```python
from build123d import *

# Parameters (mm, degrees)
F1_DEPTH = 2.2
F2_R     = 4


with BuildPart() as f1:
    # F0 (on Front) → F1 (new body)
    with BuildSketch(Plane.XZ):
        with BuildLine():
            Line((-31, 0), (31, 0))
            Line((31, 0), (31, 11.8))
            ThreePointArc((31, 11.8), (22.8, 20), (31, 28.2))
            Line((31, 28.2), (31, 42))
            Line((31, 42), (-31, 42))
            Line((-31, 42), (-31, 28.2))
            ThreePointArc((-31, 28.2), (-22.8, 20), (-31, 11.8))
            Line((-31, 11.8), (-31, 0))
        make_face()
    extrude(amount=F1_DEPTH)

    # F2
    f2_edges = [f1.edges().sort_by_distance(p)[0] for p in [
        (-31, -1.1, 11.8),
        (31, -1.1, 11.8),
        (31, -1.1, 28.2),
        (-31, -1.1, 28.2),
    ]]
    fillet(f2_edges, radius=F2_R)


solid = f1.part
```
Geometry check sheet. Reference: the model listing, model coordinates, mm. A direction names the side the tool comes from. Round coordinates to 2 decimals unless told otherwise and drop trailing zeros. Loops run counter-clockwise (first coordinate to the right, second up) from the corner with the lowest first, then second, coordinate; pieces in that order, holes last. Notation, with made-up numbers: (79.5, 82) - (120.5, 82) arc R13 cw to (120.5, 104) - close; hole circle Ø5 at (-28, 73.5). An arc over 180 degrees is marked (long way). Write item = value, one per line. Start each with the question number.
1. Mould release check, pull along Z, two halves, no side actions. Record for faces 1 (the face through (-30.279, -1.115, 29.235)), 2 (the face through (0, -1, 0)), 3 (the face through (-31, -1, 37)): released by +Z, released by -Z, zero draft, split by the parting line, or undercut.
2. Set-up check for faces 4 (the face through (-30.24, -1.12, 10.82)), 5 (the face through (30.279, -1.115, 10.765)), 6 (the face through (-31, -1, 4)): record each of +Z, -Z, +X, -X, +Y, -Y from which the full face is reachable in a straight line by a thin tool's end or side.
3. Section check C-C on z = 14. Enter the section's corners in (x, y).
4. Thickness scan on line 1 (Z direction, x = 27.5, y = -0.9); line 2 (X direction, y = -1.25, z = 14); line 3 (X direction, y = -0.35, z = 16). Record the ranges inside material, lowest first.
5. Section check D-D on z = 20.5. Enter the section's corners in (x, y), then the cut area to 3 significant figures.
6. Section check B-B on y = -1. Enter the section's corners in (x, z).
7. Section check A-A on x = 25. Enter the section's corners in (y, z), then the cut area to 3 significant figures.
Working result:
q1.face_1 = undercut
q1.face_2 = released by -Z
q1.face_3 = zero draft
q2.face_4 = -X, +Y, -Y
q2.face_5 = +X, +Y, -Y
q2.face_6 = +Z, -Z, -X, +Y, -Y
q3.outline = (-25.41, -2.2) - (25.41, -2.2) - (25.41, 0) - (-25.41, 0) - close
q4.line_1 = 0 to 12.58, 27.42 to 42
q4.line_2 = -25.41 to 25.41
q4.line_3 = -23.84 to 23.84
q5.outline = (-22.82, -2.2) - (22.82, -2.2) - (22.82, 0) - (-22.82, 0) - close
q5.area = 100 mm^2
q6.outline = (-31, 0) - (31, 0) - (31, 8.47) arc R4 ccw to (28.31, 12.25) arc R8.2 cw to (28.31, 27.75) arc R4 ccw to (31, 31.53) - (31, 42) - (-31, 42) - (-31, 31.53) arc R4 ccw to (-28.31, 27.75) arc R8.2 cw to (-28.31, 12.25) arc R4 ccw to (-31, 8.47) - close
q7.outline = (-2.2, 0) - (0, 0) - (0, 14.41) - (-2.2, 14.41) - close; (-2.2, 25.59) - (0, 25.59) - (0, 42) - (-2.2, 42) - close
q7.area = 67.8 mm^2
